Check sheet for the modelled part. Datum: model origin and axes. Units: mm. Face numbers are marked on the shaded views. A direction names the side the tool comes from. Round coordinates to 2 decimals unless told otherwise and drop trailing zeros. Order: outer loops, then holes, each group sorted by start corner. A loop starts at its lowest first (then second) coordinate and runs counter-clockwise, first axis right, second up.
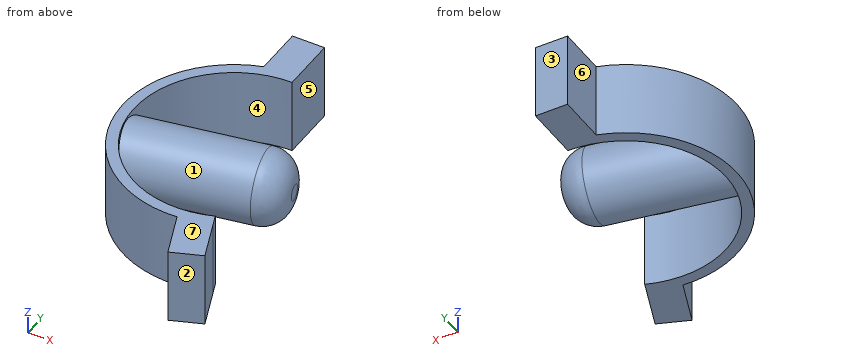
Autodesk Inventor part; units mm, degrees
ref_plane "Work Plane1" through (0, 0, 0) normal (0.1818, -0.9833, 0) x (0, 0, -1)
ref_plane "YZ Plane" through (0, 0, 0) normal (1, 0, 0) x (0, 1, 0)
ref_plane "XZ Plane" through (0, 0, 0) normal (0, 1, 0) x (-1, 0, 0)
sketch "Sketch1" plane through (0, 0, 0) normal (0, 0, 1) x (1, 0, 0)
  arc A0 (0, 12.7) -> (4.541, -11.8604) centre (0, 0) ccw
  arc A1 (0, 11.43) -> (4.0869, -10.6744) centre (0, 0) ccw
  line L0 (0, 11.43) -> (0, 12.7)
  line L1 (4.541, -11.8604) -> (4.0869, -10.6744)
  dimension "d0" = 25.4
  dimension "d1" = 22.86
extrude "Extrusion1" add sketch "Sketch1" along normal blind 8.636
ref_plane "Work Plane1" through (0, 0, 0) normal (0.1818, -0.9833, 0) x (0, 0, -1)
sketch "Sketch2" plane through (0, 0, 0) normal (0.1818, -0.9833, 0) x (0, 0, -1)
  line L0 (-8.636, -11.43) -> (0, -11.43)
  point P0 (0, 0)
  point P1 (-4.318, -11.43)
ref_plane "Work Plane2" through (-11.2395, -2.0781, 4.318) normal (0.9833, 0.1818, 0) x (-0.1818, 0.9833, 0)
sketch "Sketch3" plane through (-11.2395, -2.0781, 4.318) normal (0.9833, 0.1818, 0) x (-0.1818, 0.9833, 0)
  circle A0 centre (0, 0) radius 4.064
  point P0 (0, -4.318)
  dimension "d4" = 8.128
extrude "Extrusion2" add sketch "Sketch3" along normal blind 17.78
fillet "Fillet1" radius 3.175 1 edges at (6.983, -2.8418, 4.318)
ref_plane "Work Plane3" through (0, 12.7, 0) normal (0, 1, 0) x (-1, 0, 0)
sketch "Sketch4" plane through (0, 12.7, 0) normal (0, 1, 0) x (-1, 0, 0)
  line L0 (0, 0) -> (0, 8.636)
  line L1 (-4.0869, 8.636) -> (11.43, 8.636)
  line L2 (0, 0) -> (3.6716, 0)
  line L3 (3.6716, 0) -> (3.6716, 8.636)
  line L4 (3.6716, 8.636) -> (0, 8.636)
  line L5 (0, 8.636) -> (0, 0)
extrude "Extrusion3" add sketch "Sketch4" along normal blind 5.08 and the other way blind 0.9525
ref_plane "Work Plane4" through (4.541, -11.8604, 0) normal (0.3576, -0.9339, 0) x (0.9339, 0.3576, 0)
sketch "Sketch5" plane through (4.541, -11.8604, 0) normal (0.3576, -0.9339, 0) x (0.9339, 0.3576, 0)
  line L0 (-3.7062, 0) -> (-3.7062, 8.66)
  line L1 (-3.7062, 0) -> (0, 0)
  line L2 (0, 0) -> (0, 8.636)
  line L3 (0, 8.636) -> (-3.7062, 8.636)
  line L4 (-3.7062, 8.636) -> (-3.7062, 0)
  line L5 (0.9182, 8.636) -> (-12.7, 8.636)
  line L6 (0, 0) -> (0, 8.636)
  line L7 (0.9182, 0) -> (-12.7, 0)
  point P0 (-3.7062, 8.636)
  dimension "d12" = 0
  dimension "d13" = 0
  dimension "d14" = 0
extrude "Extrusion4" add sketch "Sketch5" along normal blind 5.08 and the other way blind 1.016
properties part number "Clip1"
1) Gauge pin test, flat ends, axial feed: pin 1 (1.7 mm diameter, centred on y = 13.5, z = 2.5, fed in from -X); pin 2 (10 mm diameter, centred on x = -4.5, y = 6.5, fed in from -Z); pin 3 (2 mm diameter, centred on x = -9.5, y = -3, fed in from +Z); pin 4 (4 mm diameter, centred on y = 12.5, z = 6.5, fed in from +X). Record the tip position at first contact, or that the pin passes through.
2) Sectioned sample at D-D on y = 5.5. Record the cut outline in (x, z).
3) Set-up check for the marked faces 5, 6 and 7: record each of +Z, -Z, +X, -X, +Y, -Y from which the full face is reachable in a straight line by a thin tool's end or side.
4) Draft check along X on the marked faces 1, 2, 3 and 4. Enter one of: pulls with the +X half, pulls with the -X half, needs draft (parallel to the pull), parting line crosses it, or undercut.
5) Scan lines: line 1 (Y direction, x = -3.5, z = 5); line 2 (Y direction, x = -5, z = 1.25); line 3 (Y direction, x = 4, z = 4.75). Record each from-to range of solid material in increasing order.
6) Sectioned sample at A-A on x = -2.5. Count the separate pieces of the cut face and the enclosed holes in it, and give its area (3 significant figures).
7) Sectioned sample at B-B on y = 12.5. Record the cut outline in (x, z), and give its area (3 significant figures).
Values found:
1. pin 1: stops at x = -3.67
1. pin 2: stops at z = 0
1. pin 3: stops at z = 8.38
1. pin 4: stops at x = 0
2. outline: (-11.45, 0) - (-10.02, 0) - (-10.02, 8.64) - (-11.45, 8.64) - close
3. face 5: +Z, -Z, +X, +Y
3. face 6: +Z, -Z, -X, +Y
3. face 7: +Z, +X, -X, +Y, -Y
4. face 1: undercut
4. face 2: pulls with the +X half
4. face 3: needs draft
4. face 4: undercut
5. line 1: y = -12.21 to -10.88, -4.72 to 3.43, 10.88 to 17.78
5. line 2: y = -11.67 to -10.28, -3.63 to 1.79, 10.28 to 11.67
5. line 3: y = -17.51 to -10.71, -3.37 to 4.43
6. separate pieces: 3
6. enclosed holes: 0
6. area: 121 mm2
7. outline: (-3.67, 0) - (0, 0) - (0, 8.64) - (-3.67, 8.64) - close
7. area: 31.7 mm2
